Geometry check sheet. Reference: the model listing, model coordinates, mm. Coordinates: 2 decimals unless noted, no trailing zeros. Write each loop counter-clockwise with the first axis right and the second up, starting at its lowest first coordinate (ties: lowest second). Pieces come first, ordered by that corner, then holes. Notation, with made-up numbers: (17, -0.75) -> (41, -0.75) arc R15 ccw to (41, 16.25) -> close; hole circle Ø2 at (-3, 80). An arc over 180 degrees is marked (long way). Answer in a Markdown table with one row per item. Add a question column.
Q1. Section check A-A, the plane z = -8.5. Record the boundary of the cut face in (x, y), and give its area (3 significant figures).
Q2. Thickness scan on line 1 (X direction, y = 1.75, z = 10); line 2 (X direction, y = 1.5, z = -10). Record the ranges inside material, lowest first.
Q3. Section check B-B, the plane x = -51. Record the boundary of the cut face in (y, z).
Q4. Gauge pin test, flat end, axial feed: P1, Ø6, axis at x = -8.5, z = -7, coming from the -Y side. Record the tip position at first contact, or that the pin passes through.
Q5. Release check for a two-part mould opening along Z. For faces 1 (the face through (-1, 2, 15)), 2 (the face through (48.56, 2.46, 9.46)), 3 (the face through (-1, 5, 0)) record: pulls with the +Z half, pulls with the -Z half, needs draft (parallel to the pull), parting line crosses it, or undercut.
```python
from build123d import *

# Parameters (mm, degrees)
SKIZZE1_W                       = 110
SKIZZE1_H                       = 30
SKIZZE1_R                       = 2.5
AUFSATZ_LINEAR_AUSTRAGEN1_DEPTH = 5


with BuildPart() as part:
    # Skizze1 → Aufsatz-Linear austragen1 (new body)
    with BuildSketch(Plane(origin=(0, 0, 0), x_dir=(1, 0, 0), z_dir=(0, 1, 0))):
        Rectangle(SKIZZE1_W, SKIZZE1_H)
        with Locations(Location((-51, 10, 0), (0, 0, 270))):
            Circle(SKIZZE1_R, mode=Mode.SUBTRACT)
        with Locations(Location((51, -10, 0), (0, 0, 270))):
            Circle(SKIZZE1_R, mode=Mode.SUBTRACT)
    extrude(amount=AUFSATZ_LINEAR_AUSTRAGEN1_DEPTH)


solid = part.part
```
Calculated:
| question | item | result |
|---|---|---|
| 1 | outline | (-55, 0) -> (-53, 0) -> (-53, 5) -> (-55, 5) -> close; (-49, 0) -> (55, 0) -> (55, 5) -> (-49, 5) -> close |
| 1 | area | 530 mm² |
| 2 | line 1 | x = -55 to 48.5, 53.5 to 55 |
| 2 | line 2 | x = -55 to -53.5, -48.5 to 55 |
| 3 | outline | (0, -15) -> (5, -15) -> (5, -12.5) -> (0, -12.5) -> close; (0, -7.5) -> (5, -7.5) -> (5, 15) -> (0, 15) -> close |
| 4 | P1 | stops at y = 0 |
| 5 | face 1 | pulls with the +Z half |
| 5 | face 2 | undercut |
| 5 | face 3 | needs draft |
